Check sheet for the modelled part. Datum: model origin and axes. Units: mm. A direction names the side the tool comes from. Coordinates: 2 decimals unless noted, no trailing zeros. Loops run counter-clockwise (first coordinate to the right, second up) from the corner with the lowest first, then second, coordinate; pieces in that order, holes last.
```python
from build123d import *

# Parameters (mm, degrees)
SKETCH1_W           = 25.5
SKETCH1_H           = 21.5
BOSS_EXTRUDE1_DEPTH = 65.5
SKETCH2_W           = 22.5
SKETCH2_H           = 18.5
CUT_EXTRUDE1_DEPTH  = 64
CUT_EXTRUDE2_DEPTH  = 21.5


with BuildPart() as part:
    # Sketch1 → Boss-Extrude1 (new body)
    with BuildSketch(Plane(origin=(0, 0, 0), x_dir=(1, 0, 0), z_dir=(0, 1, 0))):
        with Locations((-53.846079549, -25.043168737)):
            Rectangle(SKETCH1_W, SKETCH1_H)
    extrude(amount=BOSS_EXTRUDE1_DEPTH)

    # Sketch2 → Cut-Extrude1 (cut)
    with BuildSketch(Plane(origin=(0, 65.5, 0), x_dir=(1, 0, 0), z_dir=(0, 1, 0))):
        with Locations((-53.846079549, -25.043168737)):
            Rectangle(SKETCH2_W, SKETCH2_H)
    extrude(amount=-CUT_EXTRUDE1_DEPTH, mode=Mode.SUBTRACT)

    # Sketch5 → Cut-Extrude2 (cut)
    with BuildSketch(Plane.XY.offset(35.793168737)):
        with BuildLine():
            Line((-45.096079549, 65.5), (-62.596079549, 65.5))
            Line((-62.596079549, 65.5), (-62.596079549, 10))
            ThreePointArc((-62.596079549, 10), (-60.838720236, 5.757359313), (-56.596079549, 4))
            Line((-56.596079549, 4), (-51.096079549, 4))
            ThreePointArc((-51.096079549, 4), (-46.853438862, 5.757359313), (-45.096079549, 10))
            Line((-45.096079549, 10), (-45.096079549, 65.5))
        make_face()
    extrude(amount=-CUT_EXTRUDE2_DEPTH, mode=Mode.SUBTRACT)


solid = part.part
```
1) Section check D-D on y = 9. Enter the section's corners in (x, z), plus the area to 3 significant figures.
Answer sheet:
outline: (-66.6, 14.29) - (-62.51, 14.29) - (-62.51, 15.79) - (-65.1, 15.79) - (-65.1, 34.29) - (-62.51, 34.29) - (-62.51, 35.79) - (-66.6, 35.79) - close; (-45.18, 14.29) - (-41.1, 14.29) - (-41.1, 35.79) - (-45.18, 35.79) - (-45.18, 34.29) - (-42.6, 34.29) - (-42.6, 15.79) - (-45.18, 15.79) - close
area: 80.0 mm2
2) Depth check by flat-ended pin: pin 1 (2 mm diameter, centred on x = -44, z = 31, fed in from +Y). Enter the tip coordinate at first touch or a pass-through.
Answer sheet:
pin 1: stops at y = 1.5
3) Mould release check, pull along X, two halves, no side actions. Record for faces 4 (the flat face through (-44.7, 28.9, 15.793)), 5 (the flat face through (-42, 65.5, 25)): +X half, -X half, draft (parallel to the pull), parting line (faces both ways), or undercut.
Answer sheet:
face 4: undercut
face 5: draft
4) Section check C-C on z = 26.25. Enter the section's corners in (x, y), plus the area to 3 significant figures.
Answer sheet:
outline: (-66.6, 0) - (-41.1, 0) - (-41.1, 65.5) - (-42.6, 65.5) - (-42.6, 1.5) - (-65.1, 1.5) - (-65.1, 65.5) - (-66.6, 65.5) - close
area: 230 mm2
5) Scan lines: line 1 (X direction, y = 6.5, z = 16); line 2 (Z direction, x = -44.5, y = 20.5); line 3 (Y direction, x = -62, z = 26). Record each from-to range of solid material in increasing order.
Answer sheet:
line 1: x = -66.6 to -65.1, -42.6 to -41.1
line 2: z = 14.29 to 15.79, 34.29 to 35.79
line 3: y = 0 to 1.5
6) Section check A-A on y = 50. Enter the section's corners in (x, z).
Answer sheet:
outline: (-66.6, 14.29) - (-62.6, 14.29) - (-62.6, 15.79) - (-65.1, 15.79) - (-65.1, 34.29) - (-62.6, 34.29) - (-62.6, 35.79) - (-66.6, 35.79) - close; (-45.1, 14.29) - (-41.1, 14.29) - (-41.1, 35.79) - (-45.1, 35.79) - (-45.1, 34.29) - (-42.6, 34.29) - (-42.6, 15.79) - (-45.1, 15.79) - close
7) Section check B-B on x = -64.5. Enter the section's corners in (y, z), plus the area to 3 significant figures.
Answer sheet:
outline: (0, 14.29) - (65.5, 14.29) - (65.5, 15.79) - (1.5, 15.79) - (1.5, 34.29) - (65.5, 34.29) - (65.5, 35.79) - (0, 35.79) - close
area: 224 mm2
8) Set-up check for faces 1 (the flat face through (-54, 4, 15)), 2 (the flat face through (-63, 30, 35.793)), 3 (the flat face through (-65.096, 34, 25)): record each of +Z, -Z, +X, -X, +Y, -Y from which the full face is reachable in a straight line by a thin tool's end or side.
Answer sheet:
face 1: +Z, -Z, +Y
face 2: +Z, +X, -X, +Y, -Y
face 3: +Y
